Read the model definition and answer for the solid it produces. Units are mm, in the model's axes. Face numbers are marked on the shaded views. A direction names the side the tool comes from. Coordinates: 2 decimals unless noted, no trailing zeros. Write each loop counter-clockwise with the first axis right and the second up, starting at its lowest first coordinate (ties: lowest second). Pieces come first, ordered by that corner, then holes. Notation, with made-up numbers: (9, 1.5) -> (37, 1.5) arc R20 ccw to (37, 36.5) -> close; hole circle Ø9 at (43.5, 82.5). An arc over 180 degrees is marked (long way). Return JSON: item names as keys, results as strings.
from build123d import *

# Parameters (mm, degrees)
F1_DEPTH  = 258
F2_R      = 22.5
F2_R_2    = 3.25
F3_DEPTH  = 141.001
F2_R_3    = 5
F4_DEPTH  = 4
F5_R      = 4
F6_DEPTH  = 100.001
F7_R      = 3
F8_DEPTH  = 141.001
F9_SIZE2  = 3
F9_SIZE   = 3
F10_R     = 34.5
F10_R_2   = 19
F11_DEPTH = 9
F12_SIZE  = 1


with BuildPart() as f1:
    # F0 (on Front) → F1 (new body)
    with BuildSketch(Plane.XZ):
        with BuildLine():
            Line((0, 4), (0, 0))
            Line((0, 0), (96, 0))
            ThreePointArc((96, 0), (98.8284271247, 1.1715728753), (100, 4))
            Line((100, 4), (100, 137))
            ThreePointArc((100, 137), (98.8284271247, 139.8284271247), (96, 141))
            Line((96, 141), (0, 141))
            Line((0, 141), (0, 137))
            Line((0, 137), (94, 137))
            ThreePointArc((94, 137), (95.4142135624, 136.4142135624), (96, 135))
            Line((96, 135), (96, 6))
            ThreePointArc((96, 6), (95.4142135624, 4.5857864376), (94, 4))
            Line((94, 4), (0, 4))
        make_face()
    extrude(amount=F1_DEPTH)

    # F2 (on face) → F3 (cut, through all)
    with BuildSketch(Plane.XY.offset(141)):
        with Locations((50, -200.5)):
            Circle(F2_R)
        with Locations((50, -87.5)):
            Circle(F2_R_2)
        with Locations((50, -57.5)):
            Circle(F2_R)
        with Locations((20, -57.5)):
            Circle(F2_R_2)
        with Locations((80, -57.5)):
            Circle(F2_R_2)
        with Locations((50, -27.5)):
            Circle(F2_R_2)
        with Locations((50, -170.5)):
            Circle(F2_R_2)
        with Locations((80, -200.5)):
            Circle(F2_R_2)
        with Locations((50, -230.5)):
            Circle(F2_R_2)
        with Locations((20, -200.5)):
            Circle(F2_R_2)
    extrude(amount=-F3_DEPTH, mode=Mode.SUBTRACT)

    # F2 (on face) → F4 (cut, through all)
    with BuildSketch(Plane.XY.offset(141)):
        with Locations((50, -129)):
            Circle(F2_R_3)
    extrude(amount=-F4_DEPTH, mode=Mode.SUBTRACT)

    # F5 (on face) → F6 (cut, through all)
    with BuildSketch(Plane.YZ.offset(100)):
        with Locations((-233.5, 93.5)):
            Circle(F5_R)
        with Locations((-233.5, 47.5)):
            Circle(F5_R)
        with Locations((-157.5, 93.5)):
            Circle(F5_R)
        with Locations((-157.5, 47.5)):
            Circle(F5_R)
        with Locations((-100.5, 93.5)):
            Circle(F5_R)
        with Locations((-100.5, 47.5)):
            Circle(F5_R)
        with Locations((-24.5, 93.5)):
            Circle(F5_R)
        with Locations((-24.5, 47.5)):
            Circle(F5_R)
    extrude(amount=-F6_DEPTH, mode=Mode.SUBTRACT)

    # F7 (on face) → F8 (cut, through all)
    with BuildSketch(Plane.XY.offset(141)):
        with Locations((10, -239)):
            Circle(F7_R)
        with Locations((10, -19)):
            Circle(F7_R)
    extrude(amount=-F8_DEPTH, mode=Mode.SUBTRACT)

    # F9
    f9_edges = [f1.edges().sort_by_distance(p)[0] for p in [
        (7, -19, 141),
        (7, -239, 141),
        (7, -239, 0),
        (7, -19, 0),
    ]]
    chamfer(f9_edges, length=F9_SIZE, length2=F9_SIZE2)

    # F10 (on face) → F11 (join)
    with BuildSketch(Plane(origin=(0, 0, 0), x_dir=(1, 0, 0), z_dir=(0, 0, -1))):
        with Locations((50, 57.5)):
            Circle(F10_R)
        with Locations((50, 57.5)):
            Circle(F10_R_2, mode=Mode.SUBTRACT)
        with Locations((50, 200.5)):
            Circle(F10_R)
        with Locations((50, 200.5)):
            Circle(F10_R_2, mode=Mode.SUBTRACT)
    extrude(amount=F11_DEPTH)

    # F12
    f12_edges = [f1.edges().sort_by_distance(p)[0] for p in [
        (15.5, -200.5, -9),
        (15.5, -57.5, -9),
    ]]
    chamfer(f12_edges, length=F12_SIZE)


solid = f1.part
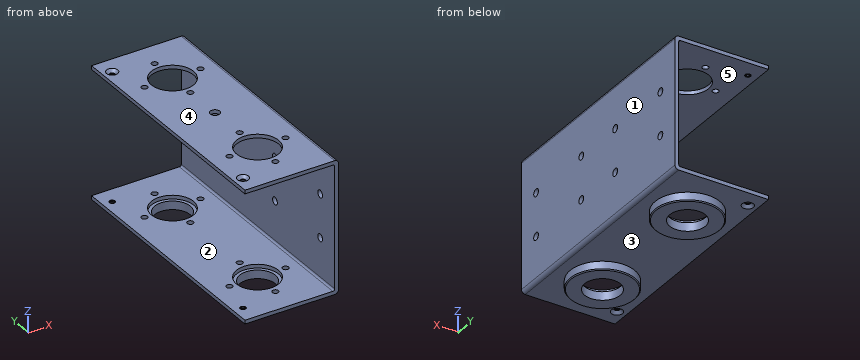
1. For a pull along Z with two mould halves and no side action, classify the marked faces 3, 4 and 5 as +Z half, -Z half, draft (parallel to the pull), parting line (faces both ways), or undercut.
Taken from the geometry:
{"face 3": "-Z half", "face 4": "+Z half", "face 5": "undercut"}
2. Flat-ended cylindrical pins translate along their axes: pin 1 Ø6 at (x, y) = (50, -87.5) entering from +Z; pin 2 Ø7 at (x, y) = (10, -239) entering from -Z; pin 3 Ø4 at (x, y) = (64.5, -49) entering from +Z; pin 4 Ø1 at (x, y) = (42, -106) entering from -Z. Find the tip coordinate at first contact, or state that the pin passes through.
Taken from the geometry:
{"pin 1": "stops at z = 0", "pin 2": "stops at z = 2.5", "pin 3": "passes through", "pin 4": "stops at z = 0"}
3. The part is cut by section C-C (y = -100). Determine the outline of the cut face in (x, z), then the cut area to 3 significant figures.
Taken from the geometry:
{"outline": "(0, 0) -> (96, 0) arc R4 ccw to (100, 4) -> (100, 43.53) -> (96, 43.53) -> (96, 6) arc R2 cw to (94, 4) -> (0, 4) -> close; (0, 137) -> (94, 137) arc R2 cw to (96, 135) -> (96, 97.47) -> (100, 97.47) -> (100, 137) arc R4 ccw to (96, 141) -> (0, 141) -> close; (96, 51.47) -> (100, 51.47) -> (100, 89.53) -> (96, 89.53) -> close", "area": "1,260 mm2"}
4. A tool of negligible diameter and unlimited length cuts with its end or side. For the marked faces 1 and 2, from which of +Z, -Z, +X, -X, +Y, -Y can it reach the whole face along a straight path? Write none if from no direction.
Taken from the geometry:
{"face 1": "+Z, -Z, +X, +Y, -Y", "face 2": "-X, +Y, -Y"}
5. Consider L1, parallel to Z at x = 16.5, y = -133; L2, parallel to Z at x = 68, y = -179.5; L3, parallel to Z at x = 98.15, y = -24.5. Determine where each line is inside the solid, lowest interval first.
Taken from the geometry:
{"L1": "z = 0 to 4, 137 to 141", "L2": "z = -9 to 4, 137 to 141", "L3": "z = 0.63 to 43.5, 51.5 to 89.5, 97.5 to 140.37"}
6. The part is cut by section B-B (z = 93.5). Determine the outline of the cut face in (x, y).
Taken from the geometry:
{"outline": "(96, -258) -> (100, -258) -> (100, -237.5) -> (96, -237.5) -> close; (96, -229.5) -> (100, -229.5) -> (100, -161.5) -> (96, -161.5) -> close; (96, -153.5) -> (100, -153.5) -> (100, -104.5) -> (96, -104.5) -> close; (96, -96.5) -> (100, -96.5) -> (100, -28.5) -> (96, -28.5) -> close; (96, -20.5) -> (100, -20.5) -> (100, 0) -> (96, 0) -> close"}
7. The part is cut by section A-A (x = 10). Count the separate pieces of the cut face and the enclosed holes in it, then the cut area to 3 significant figures.
Taken from the geometry:
{"separate pieces": "6", "enclosed holes": "0", "area": "1,930 mm2"}
